Input: dimensioned drawing with shaded views. Units: mm. Origin: part minimum x, y, z. A direction names the side the tool comes from. Round coordinates to 2 decimals unless told otherwise and drop trailing zeros. Order: outer loops, then holes, each group sorted by start corner. A loop starts at its lowest first (then second) coordinate and runs counter-clockwise, first axis right, second up. Notation, with made-up numbers: M 39,49 L 61,49 A22 ccw 61,55 Z; hole C 57,-38 d9. An arc over 180 degrees is marked long. Answer as CSV lines item,"result". Start each with the question number.
Item 1: Set-up query: the marked faces 4 and 5. Return all of +Z, -Z, +X, -X, +Y, -Y with unobstructed straight access to the full face (end or side cutting, diameter ignored); none if empty.
Item 2: Line query: line 1 (X direction, y = 2, z = 3.75) (1 decimal); line 2 (X direction, y = 4.4, z = 1.5) (1 decimal); line 3 (Y direction, x = 6.25, z = 1). Output: solid intervals per line, ascending. Write a range as [from, to].
Item 3: Section query C-C on y = 1.4. Return the cut outline in (x, z).
Item 4: Section query B-B on y = 2.3. Return the cut outline in (x, z).
Item 5: Section query A-A on x = 4. Return the cut outline in (y, z).
Item 6: Pull-direction query (X, two-part tool) for the marked faces 1, 2 and 3; classes: +X half, -X half, draft (parallel to the pull), parting line (faces both ways), or undercut.
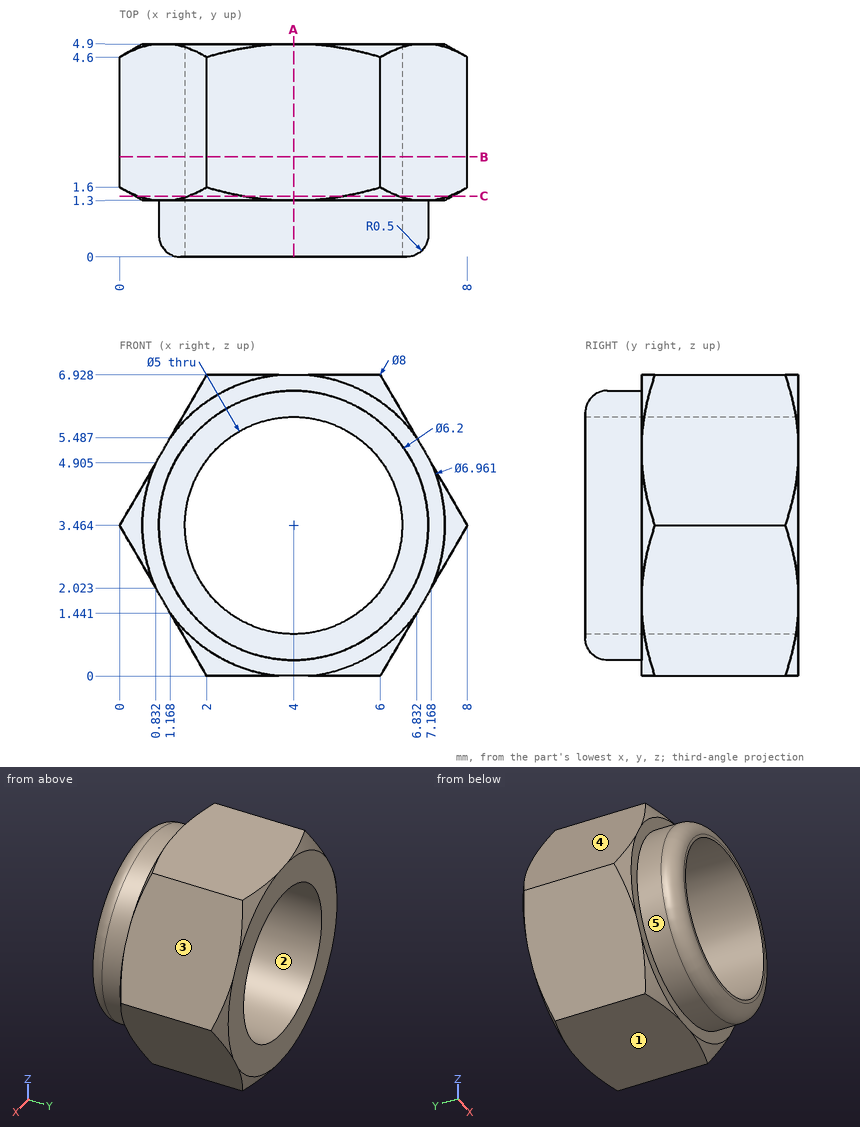
Results:
1,face 4,"+Z, -X, +Y, -Y"
1,face 5,"-Y"
2,line 1,"[0.2, 1.5], [6.5, 7.8]"
2,line 2,"[1.1, 2.5], [5.5, 6.9]"
2,line 3,"[1.3, 4.9]"
3,outline,"M 0.42,2.74 L 1.58,0.73 A3.65 ccw 2.84,0 L 5.16,0 A3.65 ccw 6.42,0.73 L 7.58,2.74 A3.65 ccw 7.58,4.19 L 6.42,6.2 A3.65 ccw 5.16,6.93 L 2.84,6.93 A3.65 ccw 1.58,6.2 L 0.42,4.19 A3.65 ccw Z; hole C 4,3.46 d5"
4,outline,"M 0,3.46 L 2,0 L 6,0 L 8,3.46 L 6,6.93 L 2,6.93 Z; hole C 4,3.46 d5"
5,outline,"M 0,0.86 A0.5 ccw 0.5,0.36 L 1.3,0.36 L 1.3,0 L 4.9,0 L 4.9,0.96 L 0,0.96 Z; M 0,5.96 L 4.9,5.96 L 4.9,6.93 L 1.3,6.93 L 1.3,6.56 L 0.5,6.56 A0.5 ccw 0,6.06 Z"
6,face 1,"draft"
6,face 2,"undercut"
6,face 3,"+X half"
